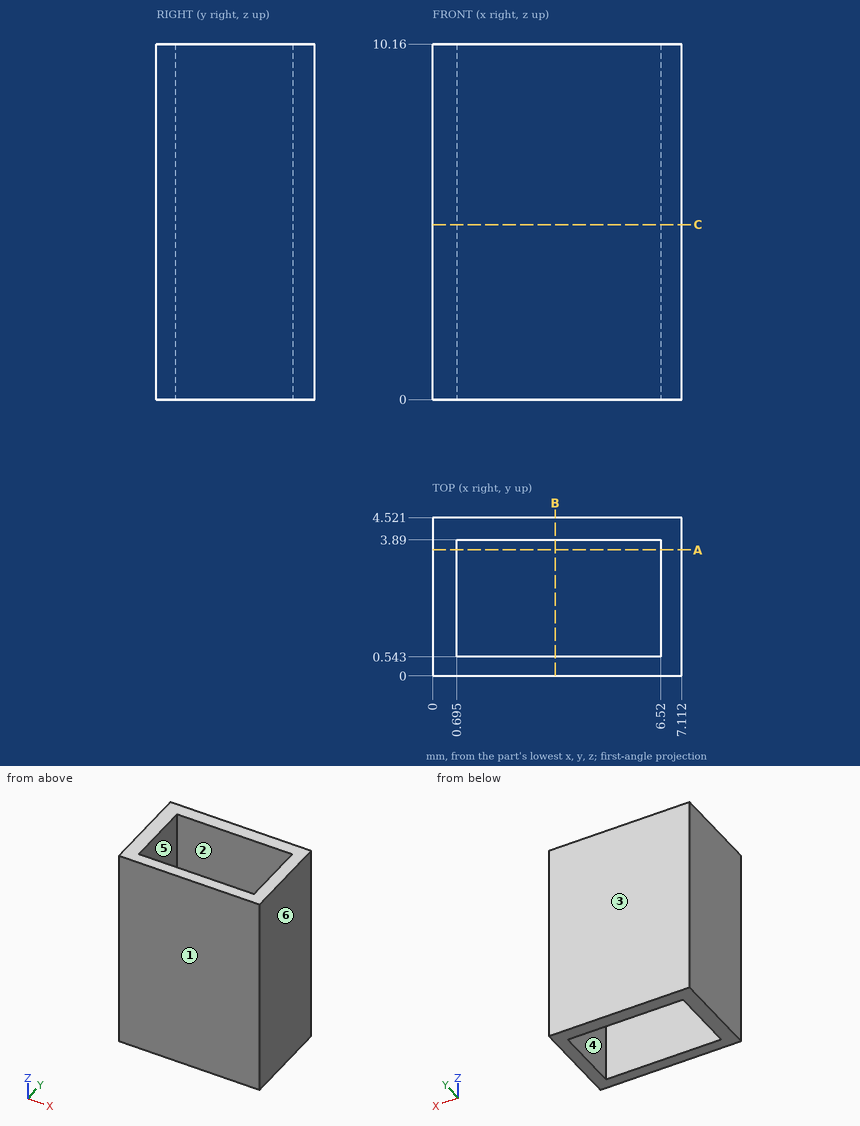
Geometry check sheet. Reference: drawing and pictorial views, mm from the part's lowest x, y, z. A direction names the side the tool comes from. Coordinates: 2 decimals unless noted, no trailing zeros. Order: outer loops, then holes, each group sorted by start corner. A loop starts at its lowest first (then second) coordinate and runs counter-clockwise, first axis right, second up.
1. Scan lines: line 1 (Y direction, x = 4.75, z = 9.25); line 2 (X direction, y = 3.45, z = 4.5) (1 decimal). Record each from-to range of solid material in increasing order.
Results found:
line 1: y = 0 to 0.54, 3.89 to 4.52
line 2: x = 0 to 0.7, 6.5 to 7.1
2. Sectioned sample at A-A, the plane y = 3.6. Record the cut outline in (x, z) (1 decimal).
Results found:
outline: (0, 0) - (0.7, 0) - (0.7, 10.2) - (0, 10.2) - close; (6.5, 0) - (7.1, 0) - (7.1, 10.2) - (6.5, 10.2) - close
3. Release check for a two-part mould opening along Y. For the marked faces 3, 4, 5 and 6 record: +Y half, -Y half, draft (parallel to the pull), parting line (faces both ways), or undercut.
Results found:
face 3: +Y half
face 4: undercut
face 5: undercut
face 6: draft
4. Sectioned sample at B-B, the plane x = 3.5. Record the cut outline in (y, z).
Results found:
outline: (0, 0) - (0.54, 0) - (0.54, 10.16) - (0, 10.16) - close; (3.89, 0) - (4.52, 0) - (4.52, 10.16) - (3.89, 10.16) - close
5. Set-up check for the marked faces 1 and 2: record each of +Z, -Z, +X, -X, +Y, -Y from which the full face is reachable in a straight line by a thin tool's end or side.
Results found:
face 1: +Z, -Z, +X, -X, -Y
face 2: +Z, -Z
6. Sectioned sample at C-C, the plane z = 5. Record the cut outline in (x, y) (1 decimal).
Results found:
outline: (0, 0) - (7.1, 0) - (7.1, 4.5) - (0, 4.5) - close; hole (0.7, 0.5) - (6.5, 0.5) - (6.5, 3.9) - (0.7, 3.9) - close
